Geometry check sheet. Reference: the model listing, model coordinates, mm. Face numbers are marked on the shaded views. A direction names the side the tool comes from. Give positions to 0.01 mm unless a question says otherwise; leave off trailing zeros. Write each loop counter-clockwise with the first axis right and the second up, starting at its lowest first coordinate (ties: lowest second). Pieces come first, ordered by that corner, then holes. Notation, with made-up numbers: (37, 68) - (58, 68) arc R19 cw to (58, 72) - close; hole circle Ø11 at (0, 31.25). An arc over 180 degrees is marked (long way). Write item = value, one per line. Start each with the question number.
(1) Depth check by flat-ended pin: pin 1 Ø8 at (x, y) = (57, 14.5) entering from +Z; pin 2 Ø13.5 at (x, z) = (30, 0) entering from -Y. Enter the tip coordinate at first touch or a pass-through.
(2) Section check C-C, the plane y = 4. Enter the section's corners in (x, z).
(3) Section check A-A, the plane x = 30. Enter the section's corners in (y, z).
(4) Access from +Z, -Z, +X, -X, +Y, -Y to the whole of each face (thin tool, end or side, straight path). Record for the marked faces 4 and 5.
(5) Section check D-D, the plane x = 0. Enter the section's corners in (y, z), plus the area to 3 significant figures.
(6) Section check B-B, the plane z = -6. Enter the section's corners in (x, y), plus the area to 3 significant figures.
(7) Thickness scan on L1, parallel to X at y = 11.5, z = 0; L2, parallel to X at y = 16.75, z = 17.5; L3, parallel to Z at x = 30, y = 9.5. Record the ranges inside material, lowest first.
(8) Draft check along X on the marked faces 1, 2 and 3. Enter one of: pulls with the +X half, pulls with the -X half, needs draft (parallel to the pull), parting line crosses it, or undercut.
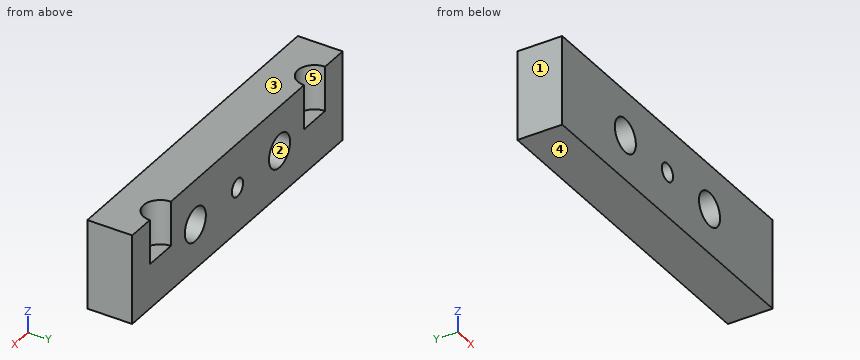
```python
from build123d import *

# Parameters (mm, degrees)
CROQUIS1_W     = 150
CROQUIS1_H     = 40
EXTRUIR1_DEPTH = 20
CROQUIS4_R     = 7.5
CROQUIS4_R_2   = 4
EXTRUIR3_DEPTH = 81.156097709
CROQUIS5_R     = 7.5
EXTRUIR4_DEPTH = 20


with BuildPart() as part:
    # Croquis1 → Extruir1 (new body)
    with BuildSketch(Plane(origin=(0, 0, 0), x_dir=(1, 0, 0), z_dir=(0, 1, 0))):
        Rectangle(CROQUIS1_W, CROQUIS1_H)
    extrude(amount=EXTRUIR1_DEPTH)

    # Croquis4 → Extruir3 (cut, through all)
    with BuildSketch(Plane(origin=(0, 20, 0), x_dir=(1, 0, 0), z_dir=(0, 1, 0))):
        with Locations(Location((-30, 0, 0), (0, 0, 270))):
            Circle(CROQUIS4_R)
        with Locations(Location((30, 0, 0), (0, 0, 90))):
            Circle(CROQUIS4_R)
        with Locations(Location((0, 0, 0), (0, 0, 270))):
            Circle(CROQUIS4_R_2)
    extrude(amount=-EXTRUIR3_DEPTH, mode=Mode.SUBTRACT)

    # Croquis5 → Extruir4 (cut)
    with BuildSketch(Plane.XY.offset(20)):
        with Locations((-55, 20)):
            Circle(CROQUIS5_R)
        with Locations((55, 20)):
            Circle(CROQUIS5_R)
    extrude(amount=-EXTRUIR4_DEPTH, mode=Mode.SUBTRACT)


solid = part.part
```
Model answer:
q1.pin_1 = 20
q1.pin_2 = through
q2.outline = (-75, -20) - (75, -20) - (75, 20) - (-75, 20) - close; hole circle Ø15 at (-30, 0); hole circle Ø8 at (0, 0); hole circle Ø15 at (30, 0)
q3.outline = (0, -20) - (20, -20) - (20, -7.5) - (0, -7.5) - close; (0, 7.5) - (20, 7.5) - (20, 20) - (0, 20) - close
q4.face_4 = -Z, +X, -X, +Y, -Y
q4.face_5 = +Z, +Y
q5.outline = (0, -20) - (20, -20) - (20, -4) - (0, -4) - close; (0, 4) - (20, 4) - (20, 20) - (0, 20) - close
q5.area = 640 mm²
q6.outline = (-75, 0) - (-34.5, 0) - (-34.5, 20) - (-75, 20) - close; (-25.5, 0) - (25.5, 0) - (25.5, 20) - (-25.5, 20) - close; (34.5, 0) - (75, 0) - (75, 20) - (34.5, 20) - close
q6.area = 2,640 mm²
q7.L1 = -75 to -37.5, -22.5 to -4, 4 to 22.5, 37.5 to 75
q7.L2 = -75 to -61.76, -48.24 to 48.24, 61.76 to 75
q7.L3 = -20 to -7.5, 7.5 to 20
q8.face_1 = pulls with the -X half
q8.face_2 = undercut
q8.face_3 = needs draft
